The model under review builds one solid part; all positions refer to its coordinate system, in mm. Face numbers are marked on the shaded views. A direction names the side the tool comes from. Give positions to 0.01 mm unless a question says otherwise; leave off trailing zeros. Order: outer loops, then holes, each group sorted by start corner. A loop starts at its lowest first (then second) coordinate and runs counter-clockwise, first axis right, second up. Notation, with made-up numbers: (21.25, -22) - (34.25, -22) arc R26 cw to (34.25, 1) - close; hole circle Ø11 at (29, -35.5). An arc over 180 degrees is marked (long way). Use CSV: the item, a comma, the result in double quotes. Start each with the question number.
1. For pin 1 (3 mm diameter, centred on x = 6, y = 15.5, fed in from +Z); pin 2 (4.5 mm diameter, centred on x = 6.5, z = 38, fed in from +Y), all flat-tipped, find the tip position at first contact; note any pin that passes through.
2. Draft analysis for pull direction X (two halves, no side actions). For the marked faces 3, 4 and 5, state which applies: released by +X, released by -X, zero draft, split by the parting line, or undercut.
3. Take a section at D-D, the plane x = 7.5. State the section outline as (y, z) points.
4. Take a section at B-B, the plane z = 31.5. State the section outline as (x, y) points, then the cut area to 3 significant figures.
5. Machinability: for the marked faces 1 and 2, which of the approach directions +Z, -Z, +X, -X, +Y, -Y give a long, thin tool a straight path to every point of the face, cutting with its end or side? Answer none if there is none.
6. Take a section at A-A, the plane y = 15. State the section outline as (x, z) points, then the cut area to 3 significant figures.
7. To check wall thickness, follow line 1 (Z direction, x = 13, y = 1.5); line 2 (Y direction, x = 7.5, z = 2.15); line 3 (Z direction, x = 11.5, y = 12.75). State the ranges of each line that lie inside material, in increasing order. Write a range as [from, to].
8. Take a section at C-C, the plane x = 13.25. State the section outline as (y, z) points.
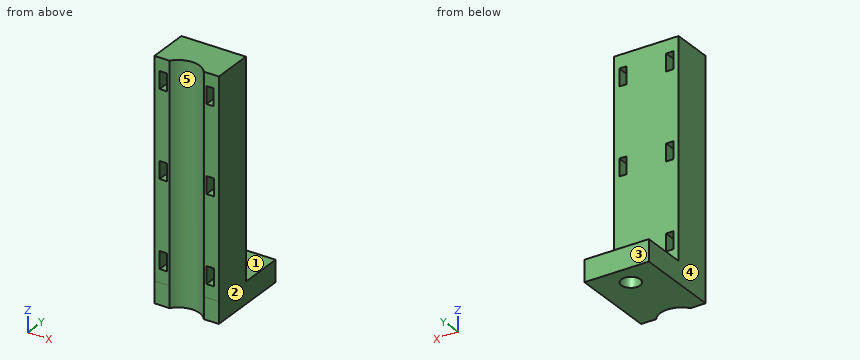
```python
from build123d import *

# Parameters (mm, degrees)
F0_W     = 15
F0_H     = 20
F0_R     = 2.2
F1_DEPTH = 5
F3_W     = 15
F3_H     = 9.501863
F4_DEPTH = 50
F5_DEPTH = 50
F6_W     = 1.7
F6_H     = 4
F7_DEPTH = 25


with BuildPart() as f1:
    # F0 (on Top) → F1 (new body)
    with BuildSketch(Plane.XY):
        with Locations((7.5, 10)):
            Rectangle(F0_W, F0_H)
        with Locations((7.5, 15)):
            Circle(F0_R, mode=Mode.SUBTRACT)
    extrude(amount=F1_DEPTH)

    # F3 (on face) → F4 (join)
    with BuildSketch(Plane.XY.offset(5)):
        with Locations((7.5, 4.750932)):
            Rectangle(F3_W, F3_H)
    extrude(amount=F4_DEPTH)

    # F2 (on face) → F5 (cut, symmetric)
    with BuildSketch(Plane.XY.offset(5)):
        with BuildLine():
            Line((3.5, 0), (11.5, 0))
            ThreePointArc((11.5, 0), (7.5, 2), (3.5, 0))
        make_face()
    extrude(amount=F5_DEPTH, both=True, mode=Mode.SUBTRACT)

    # F6 (on face) → F7 (cut)
    with BuildSketch(Plane.XZ):
        with Locations((2.05, 50)):
            Rectangle(F6_W, F6_H)
        with Locations((12.95, 50)):
            Rectangle(F6_W, F6_H)
        with Locations((2.062654, 30.000004)):
            Rectangle(F6_W, F6_H)
        with Locations((12.962654, 30.000004)):
            Rectangle(F6_W, F6_H)
        with Locations((2.075308, 10.000008)):
            Rectangle(F6_W, F6_H)
        with Locations((12.975308, 10.000008)):
            Rectangle(F6_W, F6_H)
    extrude(amount=-F7_DEPTH, mode=Mode.SUBTRACT)


solid = f1.part
```
Determined:
1,pin 1,"stops at z = 5"
1,pin 2,"stops at y = 9.5"
2,face 3,"zero draft"
2,face 4,"released by -X"
2,face 5,"undercut"
3,outline,"(2, 0) - (12.8, 0) - (12.8, 5) - (9.5, 5) - (9.5, 55) - (2, 55) - close; (17.2, 0) - (20, 0) - (20, 5) - (17.2, 5) - close"
4,outline,"(0, 0) - (1.21, 0) - (1.21, 9.5) - (0, 9.5) - close; (2.91, 0) - (3.5, 0) arc R5 cw to (11.5, 0) - (12.11, 0) - (12.11, 9.5) - (2.91, 9.5) - close; (13.81, 0) - (15, 0) - (15, 9.5) - (13.81, 9.5) - close"
4,area,"99.0 mm²"
5,face 1,"+Z, +X, -X, +Y"
5,face 2,"+Z, -Z, +X, +Y, -Y"
6,outline,"(0, 0) - (5.3, 0) - (5.3, 5) - (0, 5) - close; (9.7, 0) - (15, 0) - (15, 5) - (9.7, 5) - close"
6,area,"53.0 mm²"
7,line 1,"z = [0, 8], [12, 28], [32, 48], [52, 55]"
7,line 2,"y = [2, 12.8], [17.2, 20]"
7,line 3,"z = [0, 5]"
8,outline,"(0, 0) - (20, 0) - (20, 5) - (9.5, 5) - (9.5, 8) - (0, 8) - close; (0, 12) - (9.5, 12) - (9.5, 28) - (0, 28) - close; (0, 32) - (9.5, 32) - (9.5, 48) - (0, 48) - close; (0, 52) - (9.5, 52) - (9.5, 55) - (0, 55) - close"
